from build123d import *

# Parameters (mm, degrees)
F1_DEPTH = 50
F2_W     = 88.9
F2_H     = 63.5
F2_W_2   = 76.2
F2_H_2   = 50.8
F2_R     = 17.5
F2_W_3   = 30
F2_H_3   = 45
F3_DEPTH = 3.175
F4_W     = 442.8342580795
F4_H     = 256.8548172712
F5_DEPTH = 25.4
F6_R     = 1.27


with BuildPart() as f1:
    # F0 (on Top) → F1 (new body)
    with BuildSketch(Plane.XY):
        Polygon((33.175, -2.9), (33.175, 22.5), (33.175, 47.9), (-43.025, 47.9), (-43.025, 22.5), (-43.025, -2.9), align=None)
        with BuildLine():
            ThreePointArc((-4.85, 22.5), (-22.35, 5), (-39.85, 22.5))
            ThreePointArc((-39.85, 22.5), (-22.35, 40), (-4.85, 22.5))
        make_face(mode=Mode.SUBTRACT)
        Polygon((30, 0), (0, 0), (0, 45), (30, 45), (30, 22.5), align=None, mode=Mode.SUBTRACT)
    extrude(amount=F1_DEPTH)

    # F2 (on face) → F3 (join)
    with BuildSketch(Plane(origin=(0, 0, 0), x_dir=(1, 0, 0), z_dir=(0, 0, -1))):
        with Locations((-4.925, -22.5)):
            Rectangle(F2_W, F2_H)
        with Locations((-4.925, -22.5)):
            Rectangle(F2_W_2, F2_H_2, mode=Mode.SUBTRACT)
        with Locations((-4.925, -22.5)):
            Rectangle(F2_W_2, F2_H_2)
        with Locations((-22.35, -22.5)):
            Circle(F2_R, mode=Mode.SUBTRACT)
        with Locations((15, -22.5)):
            Rectangle(F2_W_3, F2_H_3, mode=Mode.SUBTRACT)
        with Locations((-22.35, -22.5)):
            Circle(F2_R)
        with Locations((15, -22.5)):
            Rectangle(F2_W_3, F2_H_3)
    extrude(amount=F3_DEPTH)

    # F4 (on face) → F5 (cut)
    with BuildSketch(Plane(origin=(0, 47.9, 0), x_dir=(-1, 0, 0), z_dir=(0, 1, 0))):
        with Locations((25.4539847374, 21.782644093)):
            Rectangle(F4_W, F4_H)
    extrude(amount=F5_DEPTH, mode=Mode.SUBTRACT)

    # F6
    f6_edges = [f1.edges().sort_by_distance(p)[0] for p in [
        (0, 22.5, 50),
        (33.175, 22.5, 50),
        (-4.925, 47.9, 50),
        (-43.025, 22.5, 50),
        (-4.925, -2.9, 50),
        (-39.85, 22.5, 50),
        (15, 0, 50),
        (15, 45, 50),
        (30, 22.5, 50),
    ]]
    fillet(f6_edges, radius=F6_R)


solid = f1.part
Build history of the part. All positions in model axes, mm. A direction names the side the tool comes from. Give positions to 0.01 mm unless a question says otherwise; leave off trailing zeros. Write each loop counter-clockwise with the first axis right and the second up, starting at its lowest first coordinate (ties: lowest second). Pieces come first, ordered by that corner, then holes. Notation, with made-up numbers: (-0.5, 77.25) - (19.5, 77.25) arc R13 ccw to (19.5, 96.25) - close; hole circle Ø3 at (49.25, -27). An arc over 180 degrees is marked (long way). Use one line per item in the form item = value. Start each with the question number.
1. Band-saw the part on A-A on x = 1. Write the cut outline in (y, z) (3 decimals), plus the area to 3 significant figures.
2. Band-saw the part on C-C on z = 12. Write the cut outline in (x, y) (3 decimals).
3. Two-plate mould, pull along Y, no slides. Class faces 6 (the face through (-4, 47.9, 23)), 7 (the face through (33.175, 22, 24)), 8 (the face through (30, 23, 24)): released by +Y, released by -Y, zero draft, split by the parting line, or undercut.
4. 3-axis set-ups, long thin cutter, end or side, ignore diameter. For faces 1 (the face through (-5, -4, 0)), 2 (the face through (-43.025, 23, 24)), 3 (the face through (0, 22, 24)), 4 (the face through (-5, -2.9, 24)), 5 (the face through (-6, -9.25, -2)): which of +Z, -Z, +X, -X, +Y, -Y reach the whole face in a straight line?
5. Probe line 1 (X direction, y = 22, z = 35) (3 decimals); line 2 (Y direction, x = -22.35, z = 29); line 3 (X direction, y = 29.5, z = 10) (3 decimals). List the from-to ranges inside material, lowest first. Write a range as [from, to].
6. Drop flat-ended pins along their axis: pin 1 Ø10 at (y, z) = (37.5, 24) entering from -X (3 decimals); pin 2 Ø1 at (y, z) = (27.5, 44.5) entering from +X (3 decimals); pin 3 Ø8 at (x, z) = (-25.5, 44) entering from -Y. Give the stop position or say it passes through.
7. Band-saw the part on D-D on x = -22.35. Write the cut outline in (y, z) (3 decimals).
8. Band-saw the part on B-B on y = 22.5. Write the cut outline in (x, z) (3 decimals), plus the area to 3 significant figures.
Conclusion:
q1.outline = (-9.25, -3.175) - (47.9, -3.175) - (47.9, 48.73) arc R1.27 ccw to (46.63, 50) - (46.27, 50) arc R1.27 ccw to (45, 48.73) - (45, 0) - (0, 0) - (0, 48.73) arc R1.27 ccw to (-1.27, 50) - (-1.63, 50) arc R1.27 ccw to (-2.9, 48.73) - (-2.9, 0) - (-9.25, 0) - close
q1.area = 470 mm²
q2.outline = (-43.025, -2.9) - (33.175, -2.9) - (33.175, 47.9) - (-43.025, 47.9) - close; hole circle Ø35 at (-22.35, 22.5); hole (0, 0) - (30, 0) - (30, 45) - (0, 45) - close
q3.face_6 = released by +Y
q3.face_7 = zero draft
q3.face_8 = undercut
q4.face_1 = +Z, -Y
q4.face_2 = +Z, -X, +Y, -Y
q4.face_3 = +Z
q4.face_4 = +Z, +X, -X, -Y
q4.face_5 = +Z, -Z, +X, -X, -Y
q5.line_1 = [-43.025, -39.843], [-4.857, 0], [30, 33.175]
q5.line_2 = [-2.9, 5], [40, 47.9]
q5.line_3 = [-43.025, -38.389], [-6.311, 0], [30, 33.175]
q6.pin_1 = -43.025
q6.pin_2 = 33.175
q6.pin_3 = -2.9
q7.outline = (-9.25, -3.175) - (47.9, -3.175) - (47.9, 48.73) arc R1.27 ccw to (46.63, 50) - (41.27, 50) arc R1.27 ccw to (40, 48.73) - (40, 0) - (5, 0) - (5, 48.73) arc R1.27 ccw to (3.73, 50) - (-1.63, 50) arc R1.27 ccw to (-2.9, 48.73) - (-2.9, 0) - (-9.25, 0) - close
q8.outline = (-49.375, -3.175) - (39.525, -3.175) - (39.525, 0) - (33.175, 0) - (33.175, 48.73) arc R1.27 ccw to (31.905, 50) - (31.27, 50) arc R1.27 ccw to (30, 48.73) - (30, 0) - (0, 0) - (0, 48.73) arc R1.27 ccw to (-1.27, 50) - (-3.58, 50) arc R1.27 ccw to (-4.85, 48.73) - (-4.85, 0) - (-39.85, 0) - (-39.85, 48.73) arc R1.27 ccw to (-41.12, 50) - (-41.755, 50) arc R1.27 ccw to (-43.025, 48.73) - (-43.025, 0) - (-49.375, 0) - close
q8.area = 840 mm²
